Check sheet for the modelled part. Datum: model origin and axes. Units: mm. Face numbers are marked on the shaded views. A direction names the side the tool comes from. Round coordinates to 2 decimals unless told otherwise and drop trailing zeros. Order: outer loops, then holes, each group sorted by start corner. A loop starts at its lowest first (then second) coordinate and runs counter-clockwise, first axis right, second up.
(1) Tool access check on the marked faces 4, 5 and 6. Record the directions out of +Z, -Z, +X, -X, +Y, -Y that give a thin tool (end or side, any length) a straight path to the whole face; none if there is none.
(2) Mould release check, pull along Z, two halves, no side actions. Record for the marked faces 1, 2 and 3: released by +Z, released by -Z, zero draft, split by the parting line, or undercut.
(3) Depth check by flat-ended pin: pin 1 (1 mm diameter, centred on x = -2, y = 4, fed in from +Z); pin 2 (0.9 mm diameter, centred on x = -1, y = 4.5, fed in from -Z). Enter the tip coordinate at first touch or a pass-through.
(4) Thickness scan on probe 1 along Y at (x, z) = (-2.75, 2); probe 2 along Z at (x, y) = (-1.95, 7.25); probe 3 along Z at (x, y) = (-0.05, 2). Record the ranges inside material, lowest first.
(5) Sectioned sample at D-D, the plane y = 2.5. Enter the section's corners in (x, z).
(6) Sectioned sample at A-A, the plane x = -2.8. Enter the section's corners in (y, z), and give its area (3 significant figures).
(7) Sectioned sample at C-C, the plane z = -0.5. Enter the section's corners in (x, y), and give its area (3 significant figures).
(8) Sectioned sample at B-B, the plane y = 5. Enter the section's corners in (x, z) (3 decimals).
```python
from build123d import *

# Parameters (mm, degrees)
SKETCH1_W           = 20
SKETCH1_H           = 3
EXTRUDE_THIN1_DEPTH = 3
SNAP_START          = -3
SNAP_HOOK1_DEPTH    = 3
FILLET2_R           = 3


# Read off the part's stored shape, not the designer's step: Snap Hook1
with BuildPart() as part:
    # Sketch1 → Extrude-Thin1 (new body)
    with BuildSketch(Plane(origin=(0, 0, 0), x_dir=(0, 0, -1), z_dir=(1, 0, 0))):
        Rectangle(SKETCH1_W, SKETCH1_H)
    extrude(amount=-EXTRUDE_THIN1_DEPTH)

    # Snap Hook1 outline → Snap Hook1 (add)
    with BuildSketch(Plane.YZ.offset(SNAP_START)):
        Polygon((7.5, 10), (1.5, 10), (1.5, 7), (9.5, 9), (9.5, 10), (8, 10.327), (7.5, 10.327), align=None)
    snap_hook1 = extrude(amount=SNAP_HOOK1_DEPTH)

    # Mirror2: Snap Hook1 across plane
    add(snap_hook1.mirror(Plane.XY))

    # Fillet2
    fillet2_edges = [part.edges().sort_by_distance(p)[0] for p in [
        (-1.5, 1.5, 7),
        (-1.5, 1.5, -7),
        (-1.5, -1.5, 10),
        (-1.5, -1.5, -10),
    ]]
    fillet(fillet2_edges, radius=FILLET2_R)


solid = part.part
```
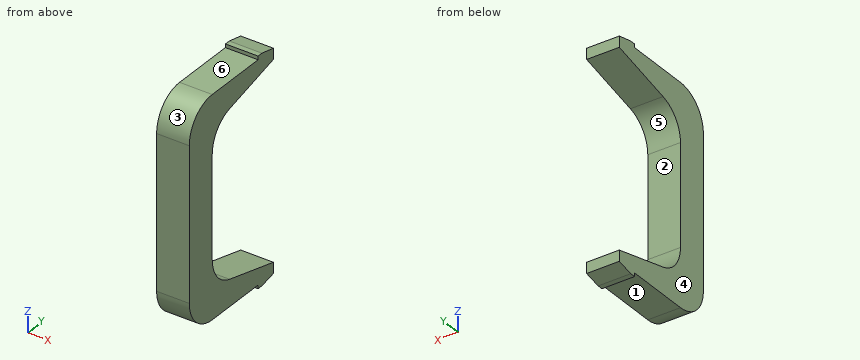
Derived:
1. face 4: +Z, -Z, -X, +Y, -Y
1. face 5: +X, -X, +Y
1. face 6: +Z, +X, -X, -Y
2. face 1: released by -Z
2. face 2: undercut
2. face 3: released by +Z
3. pin 1: stops at z = 10
3. pin 2: stops at z = -10
4. probe 1: y = -1.5 to 1.5
4. probe 2: z = -10 to -8.44, 8.44 to 10
4. probe 3: z = -10 to -6.32, 6.32 to 10
5. outline: (-3, -10) - (0, -10) - (0, -6.89) - (-3, -6.89) - close; (-3, 6.89) - (0, 6.89) - (0, 10) - (-3, 10) - close
6. outline: (-1.5, -7) arc R3 ccw to (1.5, -10) - (7.5, -10) - (7.5, -10.33) - (8, -10.33) - (9.5, -10) - (9.5, -9) - (3.77, -7.57) arc R3 cw to (1.5, -4.66) - (1.5, 4.66) arc R3 cw to (3.77, 7.57) - (9.5, 9) - (9.5, 10) - (8, 10.33) - (7.5, 10.33) - (7.5, 10) - (1.5, 10) arc R3 ccw to (-1.5, 7) - close
6. area: 91.1 mm2
7. outline: (-3, -1.5) - (0, -1.5) - (0, 1.5) - (-3, 1.5) - close
7. area: 9.00 mm2
8. outline: (-3, -10) - (0, -10) - (0, -7.875) - (-3, -7.875) - close; (-3, 7.875) - (0, 7.875) - (0, 10) - (-3, 10) - close
